Could you check a few things on this model? Use its own coordinates, in mm. A direction names the side the tool comes from. Coordinates: 2 decimals unless noted, no trailing zeros. Order: outer loops, then holes, each group sorted by start corner. A loop starts at its lowest first (then second) coordinate and runs counter-clockwise, first axis right, second up. Notation, with made-up numbers: M 39.5,27 L 48.5,27 A13 ccw 48.5,51 Z; hole C 79.25,65 d7. An arc over 180 degrees is marked long. Write item = value, one per line. Start each with the question number.
from build123d import *

# Parameters (mm, degrees)
F0_W     = 14.05
F0_H     = 92.75
F1_DEPTH = 2.94
F2_W     = 1.05
F2_H     = 92.75
F3_DEPTH = 0.5
F4_R     = 1.478073
F5_DEPTH = 2.941


with BuildPart() as f1:
    # F0 (on Top) → F1 (new body)
    with BuildSketch(Plane.XY):
        with Locations((7.025, 46.375)):
            Rectangle(F0_W, F0_H)
    extrude(amount=F1_DEPTH)

    # F2 (on face) → F3 (join)
    with BuildSketch(Plane.XY.offset(2.94)):
        with Locations((0.525, 46.375)):
            Rectangle(F2_W, F2_H)
        with Locations((13.525, 46.375)):
            Rectangle(F2_W, F2_H)
    extrude(amount=F3_DEPTH)

    # F4 (on face) → F5 (cut, through all)
    with BuildSketch(Plane.XY.offset(2.94)):
        with BuildLine():
            Line((5.546927, 45.804492), (5.546927, 37.435508))
            ThreePointArc((5.546927, 37.435508), (7.056423, 35.880334), (8.498534, 37.498191))
            Line((8.498534, 37.498191), (8.498534, 46.018191))
            ThreePointArc((8.498534, 46.018191), (6.918126, 47.356136), (5.546927, 45.804492))
        make_face()
        with Locations((7.025, 87.15)):
            Circle(F4_R)
        with Locations((7.025, 77.23)):
            Circle(F4_R)
        with Locations((7.025, 67.33)):
            Circle(F4_R)
        with Locations((7.025, 57.24)):
            Circle(F4_R)
        with Locations((7.025, 7)):
            Circle(F4_R)
        with Locations((7.025, 17)):
            Circle(F4_R)
        with Locations((7.025, 27)):
            Circle(F4_R)
    extrude(amount=-F5_DEPTH, mode=Mode.SUBTRACT)


solid = f1.part
(1) Will this pin go through, and if not, where does the flat tip stop? P1, Ø4, axis at x = 7.025, y = 27, coming from the +Z side.
(2) Imagine slicing it at A-A on y = 27. List the corners of the cut face in (x, z) for me, plus the area to 3 significant figures.
(3) Please list where these lines run through material, in increasing order: probe 1 along X at (y, z) = (39.5, 2.6); probe 2 along X at (y, z) = (79, 3.25); probe 3 along Z at (x, y) = (6, 85.5). Write a range as from..to.
(4) Imagine slicing it at C-C on x = 4. List the corners of the cut face in (y, z) for me, plus the area to 3 significant figures.
(5) Thinking about a two-plate mould opening in X: for faces 4 (the cylindrical face through (8.435, 7.444, 1.491)), 5 (the flat face through (0, 46, 2)), 6 (the flat face through (7, 0, 2)), which applies, released by +X, released by -X, zero draft, split by the parting line, or undercut?
(6) For faces 1 (the flat face through (5, 47, 0)), 2 (the flat face through (5.6, 47, 2.94)), 3 (the cylindrical face through (7.02, 35.88, 1.49)), which set-ups out of +Z, -Z, +X, -X, +Y, -Y let a thin tool reach every point of the face, with its end or its side?
Response:
q1.P1 = 2.94
q2.outline = M 0,0 L 5.55,0 L 5.55,2.94 L 1.05,2.94 L 1.05,3.44 L 0,3.44 Z; M 8.5,0 L 14.05,0 L 14.05,3.44 L 13,3.44 L 13,2.94 L 8.5,2.94 Z
q2.area = 33.7 mm2
q3.probe_1 = 0..5.55, 8.5..14.05
q3.probe_2 = 0..1.05, 13..14.05
q3.probe_3 = 0..2.94
q4.outline = M 0,0 L 92.75,0 L 92.75,2.94 L 0,2.94 Z
q4.area = 273 mm2
q5.face_4 = undercut
q5.face_5 = released by -X
q5.face_6 = zero draft
q6.face_1 = -Z, +X, -X, +Y, -Y
q6.face_2 = +Z, +Y, -Y
q6.face_3 = +Z, -Z
